Part print with two shaded views. Sizes in mm from the minimum x, y, z corner. Coordinates: 2 decimals unless noted, no trailing zeros. Write each loop counter-clockwise with the first axis right and the second up, starting at its lowest first coordinate (ties: lowest second). Pieces come first, ordered by that corner, then holes. Notation, with made-up numbers: (35.25, 57.5) - (42.25, 57.5) arc R34 ccw to (42.25, 96.5) - close; hole circle Ø8 at (-38.5, 21). An arc over 180 degrees is marked (long way). One line per question, with ' | ' between items. Start each with the question number.
1. Band-saw the part on C-C, the plane z = 0.5. Write the cut outline in (x, y), then the cut area to 3 significant figures.
2. Band-saw the part on A-A, the plane y = 3.5. Write the cut outline in (x, z).
3. Probe line 1 (Y direction, x = 3.5, z = 3.5); line 2 (Y direction, x = 4.25, z = 3.5). List the from-to ranges inside material, lowest first.
4. Band-saw the part on B-B, the plane x = 4.25. Write the cut outline in (y, z).
5. Two-plate mould, pull along X, no slides. Class the marked faces 1, 2 and 3: +X half, -X half, draft (parallel to the pull), parting line (faces both ways), or undercut.
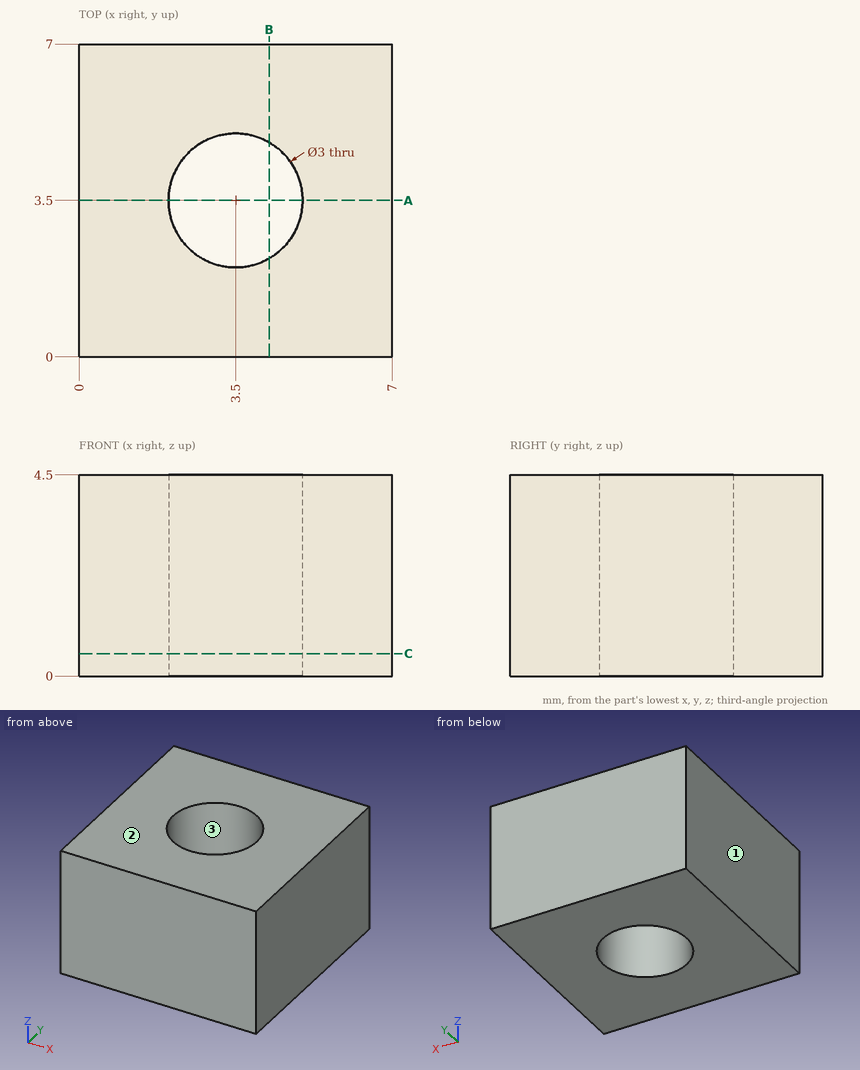
Filled in:
1) outline: (0, 0) - (7, 0) - (7, 7) - (0, 7) - close; hole circle Ø3 at (3.5, 3.5) | area: 41.9 mm²
2) outline: (0, 0) - (2, 0) - (2, 4.5) - (0, 4.5) - close; (5, 0) - (7, 0) - (7, 4.5) - (5, 4.5) - close
3) line 1: y = 0 to 2, 5 to 7 | line 2: y = 0 to 2.2, 4.8 to 7
4) outline: (0, 0) - (2.2, 0) - (2.2, 4.5) - (0, 4.5) - close; (4.8, 0) - (7, 0) - (7, 4.5) - (4.8, 4.5) - close
5) face 1: -X half | face 2: draft | face 3: undercut
